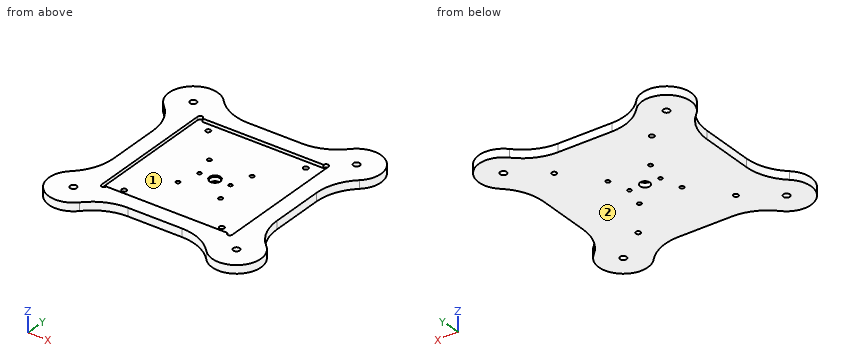
Autodesk Inventor part; units mm, degrees
ref_plane "YZ Plane" through (0, 0, 0) normal (1, 0, 0) x (0, 1, 0)
ref_plane "XZ Plane" through (0, 0, 0) normal (0, 1, 0) x (-1, 0, 0)
ref_plane "XY Plane" through (0, 0, 0) normal (0, 0, 1) x (1, 0, 0)
sketch "スケッチ1" plane through (0, 0, 0) normal (0, 0, 1) x (1, 0, 0)
  line L0 (-50, 50) -> (50, 50)
  line L1 (50, 50) -> (50, -50)
  line L2 (50, -50) -> (-50, -50)
  line L3 (-50, -50) -> (-50, 50)
  point P0 (0, 0)
  dimension "d0" = 100
  dimension "d1" = 100
  dimension "d2" = 50
  dimension "d3" = 50
extrude "押し出し1" add sketch "スケッチ1" along normal blind 3
sketch "スケッチ2" plane through (0, 0, 3) normal (0, 0, 1) x (1, 0, 0)
  point P0 (0, 0)
  point P1 (0, 0)
hole "Hole1" at (0, 0, 3) direction (0, 0, -1) diameter 6 end through all counterbore diameter 7 counterbore depth 0.5
sketch "スケッチ3" plane through (0, 0, 3) normal (0, 0, 1) x (1, 0, 0)
  circle A0 centre (0, 0) radius 3.5
  line L0 (50, 50) -> (50, -50)
  line L1 (-50, 50) -> (50, 50)
  line L2 (-50, -50) -> (-50, 50)
  line L3 (50, -50) -> (-50, -50)
  line L4 (-40.1, 40.1) -> (40.1, 40.1)
  line L5 (40.1, 40.1) -> (40.1, -40.1)
  line L6 (40.1, -40.1) -> (-40.1, -40.1)
  line L7 (-40.1, -40.1) -> (-40.1, 40.1)
  dimension "d13" = 80.2
  dimension "d14" = 80.2
  dimension "d15" = 40.1
  dimension "d16" = 40.1
extrude "押し出し2" add sketch "スケッチ3" along normal blind 2 contours L0 L3 L2 L1
sketch "スケッチ4" plane through (0, 0, 3) normal (0, 0, 1) x (1, 0, 0)
  circle A0 centre (0, 0) radius 3.5
  point P0 (-29.9, 35)
  point P1 (-29.9, -35)
  point P2 (29.9, -35)
  point P3 (29.9, 35)
  dimension "d19" = 59.8
  dimension "d20" = 59.8
  dimension "d21" = 70
  dimension "d22" = 70
  dimension "d23" = 29.9
  dimension "d24" = 29.9
  dimension "d25" = 35
hole "Hole2" at (29.9, -35, 3) at (-29.9, -35, 3) at (29.9, 35, 3) at (-29.9, 35, 3) direction (0, 0, -1) diameter 3 depth 8 tip angle 118
sketch "スケッチ5" plane through (0, 0, 0) normal (0, 0, -1) x (-1, 0, 0)
  circle A0 centre (-50, -50) radius 15
  circle A1 centre (-50, 50) radius 15
  circle A2 centre (50, -50) radius 15
  circle A3 centre (50, 50) radius 15
  dimension "d33" = 30
  dimension "d34" = 30
  dimension "d35" = 30
  dimension "d36" = 30
extrude "押し出し3" add sketch "スケッチ5" against normal blind 5
fillet "フィレット1" radius 30 8 edges at (-35, 50, 2.5) (-50, 35, 2.5) (35, 50, 2.5) (50, 35, 2.5) (50, -35, 2.5) (35, -50, 2.5) (-35, -50, 2.5) (-50, -35, 2.5)
sketch "スケッチ6" plane through (0, 0, 0) normal (0, 0, -1) x (-1, 0, 0)
  arc A0 (60, 38.8197) -> (38.8197, 60) centre (50, 50) ccw
  arc A1 (-38.8197, 60) -> (-60, 38.8197) centre (-50, 50) ccw
  arc A2 (-60, -38.8197) -> (-38.8197, -60) centre (-50, -50) ccw
  arc A3 (38.8197, -60) -> (60, -38.8197) centre (50, -50) ccw
hole "Hole3" at (-50, -50, 0) at (50, -50, 0) at (50, 50, 0) at (-50, 50, 0) direction (0, 0, 1) diameter 4 depth 8 tip angle 118
sketch "スケッチ7" plane through (0, 0, 5) normal (0, 0, 1) x (1, 0, 0)
  arc A0 (-38.731, -40.1) -> (-40.1, -38.731) centre (-50, -50) ccw
  line L0 (-40.1, -38.731) -> (-40.1, 38.731)
  arc A1 (-40.1, 38.731) -> (-38.731, 40.1) centre (-50, 50) ccw
  line L1 (-38.731, 40.1) -> (38.731, 40.1)
  arc A2 (38.731, 40.1) -> (40.1, 38.731) centre (50, 50) ccw
  line L2 (40.1, 38.731) -> (40.1, -38.731)
  arc A3 (40.1, -38.731) -> (38.731, -40.1) centre (50, -50) ccw
  line L3 (38.731, -40.1) -> (-38.731, -40.1)
  circle A4 centre (-38.6, 40.1) radius 1.5
  line L4 (38.731, 40.1) -> (-38.731, 40.1)
  line L5 (0, 40.1) -> (0, -40.1)
  line L6 (40.1, 0) -> (-40.1, 0)
  circle A5 centre (38.6, 40.1) radius 1.5
  circle A6 centre (-38.6, -40.1) radius 1.5
  circle A7 centre (38.6, -40.1) radius 1.5
  line L7 (-40.1, 40.1) -> (40.1, 40.1)
  line L8 (40.1, 40.1) -> (40.1, -40.1)
  line L9 (40.1, -40.1) -> (-40.1, -40.1)
  line L10 (-40.1, -40.1) -> (-40.1, 40.1)
  point P0 (0, 0)
  dimension "d47" = 3
  dimension "d48" = 1.5
extrude "押し出し4" cut sketch "スケッチ7" against normal up to surface (2 mm away) contours L9 A6 A0 | A0 A6 L3 | L3 A6 L9 | A6 L10 A0 | A7 A3 L3 | L3 L9 A7 | L10 A4 A1 | A3 A7 L9 | A3 L8 A7 | A4 L7 A1 | A1 L1 A4 | A4 L1 L7 | A5 L7 L1 | L1 A2 A5 | A2 A5 L8 | L7 A5 A2
sketch "スケッチ8" plane through (0, 0, 0) normal (0, 0, -1) x (-1, 0, 0)
  circle A0 centre (0, 0) radius 3
  circle A1 centre (0, 0) radius 9.5
  point P0 (-9.5, 0)
  point P1 (9.5, 0)
  dimension "d51" = 19
hole "Hole4" at (9.5, 0, 0) at (-9.5, 0, 0) direction (0, 0, 1) diameter 2.3 depth 8 tip angle 118
sketch "スケッチ9" plane through (0, 0, 0) normal (0, 0, -1) x (-1, 0, 0)
  circle A0 centre (0, 0) radius 3
  line L0 (-16.459, -50) -> (16.459, -50)
  circle A1 centre (0, 0) radius 18.5
  line L1 (0, 0) -> (13.0815, 13.0815)
  line L2 (18.5, 0) -> (0, 0)
  point P0 (-13.0815, 13.0815)
  point P1 (-13.0815, -13.0815)
  point P2 (13.0815, -13.0815)
  dimension "d59" = 37
  dimension "d60" = 45
  dimension "d63" = 360
hole "Hole5" at (-13.0815, 13.0815, 0) at (13.0815, 13.0815, 0) at (13.0815, -13.0815, 0) at (-13.0815, -13.0815, 0) direction (0, 0, 1) diameter 2.5 depth 8 tip angle 118
equation "\"d1\" = d0"
equation "\"d14\" = d13"
equation "\"d15\" = 0.5 * d13"
equation "\"d16\" = d15"
equation "\"d34\" = d33"
equation "\"d35\" = d33"
equation "\"d36\" = d33"
properties part number "JointA0"
Here's how the part is built. I have some questions about the finished solid (model axes, mm). Face numbers are marked on the shaded views. Round coordinates to 2 decimals unless told otherwise and drop trailing zeros. Loops run counter-clockwise (first coordinate to the right, second up) from the corner with the lowest first, then second, coordinate; pieces in that order, holes last. Notation, with made-up numbers: M 24,63.5 L 35,63.5 A11 cw 35,81.5 Z; hole C 60.25,-30.5 d2. An arc over 180 degrees is marked long. Write each question's results on one line, items separated by ' | '. Start each with the question number.
(1) I want a section at B-B (y = 9). Please give me the cut outline in (x, z).
(2) I want a section at C-C (y = -35). Please give me the cut outline in (x, z), then the cut area to 3 significant figures.
(3) If I drill on probe 1 along X at (y, z) = (0, 2.15); probe 2 along Y at (x, z) = (0, 1.35); probe 3 along Y at (x, z) = (-29.9, 1.4), over which ranges is the centre line in solid material (lowest first)? Write a range as from..to.
(4) Thinking about a two-plate mould opening in Y: for the marked faces 1 and 2, which applies, pulls with the +Y half, pulls with the -Y half, needs draft (parallel to the pull), parting line crosses it, or undercut?
(5) I want a section at A-A (z = 4.15). Please give me the cut outline in (x, y).
(6) Will these pins go through, and if not, where does the flat tip stop? P1, Ø1, axis at y = 32.5, z = 1.5, coming from the +X side; P2, Ø0.6, axis at y = -6, z = 4, coming from the -X side; P3, Ø1, axis at x = -5, y = 30.5, coming from the +Z side.
(7) I want a section at D-D (x = 57). Please give me the cut outline in (y, z), then the cut area to 3 significant figures.
Solved:
1) outline: M -50,0 L 50,0 L 50,5 L 40.1,5 L 40.1,3 L -40.1,3 L -40.1,5 L -50,5 Z
2) outline: M -56.42,0 L -31.4,0 L -31.4,3 L -40.1,3 L -40.1,5 L -56.42,5 Z; M -28.4,0 L 28.4,0 L 28.4,3 L -28.4,3 Z; M 31.4,0 L 56.42,0 L 56.42,5 L 40.1,5 L 40.1,3 L 31.4,3 Z | area: 386 mm²
3) probe 1: x = -50..-10.65, -8.35..-3, 3..8.35, 10.65..50 | probe 2: y = -50..-3, 3..50 | probe 3: y = -53.18..-36.5, -33.5..33.5, 36.5..53.18
4) face 1: undercut | face 2: needs draft
5) outline: M -60,-38.82 A15 ccw long -38.82,-60 A30 cw -16.46,-50 L 16.46,-50 A30 cw 38.82,-60 A15 ccw long 60,-38.82 A30 cw 50,-16.46 L 50,16.46 A30 cw 60,38.82 A15 ccw long 38.82,60 A30 cw 16.46,50 L -16.46,50 A30 cw -38.82,60 A15 ccw long -60,38.82 A30 cw -50,16.46 L -50,-16.46 A30 cw Z; hole C -50,-50 d4; hole C -50,50 d4; hole M -40.1,-40.1 A1.5 ccw -37.1,-40.1 L 37.1,-40.1 A1.5 ccw 40.1,-40.1 L 40.1,40.1 A1.5 ccw 37.1,40.1 L -37.1,40.1 A1.5 ccw -40.1,40.1 Z; hole C 50,-50 d4; hole C 50,50 d4
6) P1: stops at x = 54.97 | P2: stops at x = -50 | P3: stops at z = 3
7) outline: M -63.27,0 L -35.72,0 L -35.72,5 L -63.27,5 Z; M 35.72,0 L 63.27,0 L 63.27,5 L 35.72,5 Z | area: 275 mm²
